from build123d import *

# Parameters (mm, degrees)
SKETCH1_W           = 74.93
SKETCH1_H           = 34.036
BOSS_EXTRUDE1_DEPTH = 16.002
FILLET1_R           = 9.525
SKETCH2_R           = 2.54
BOSS_EXTRUDE2_DEPTH = 25.4
FILLET2_R           = 2.6035


with BuildPart() as part:
    # Sketch1 → Boss-Extrude1 (new body)
    with BuildSketch(Plane.XY):
        with Locations((37.465, 17.018)):
            Rectangle(SKETCH1_W, SKETCH1_H)
    extrude(amount=BOSS_EXTRUDE1_DEPTH)

    # Fillet1
    # the kernel refuses this fillet: 9.525 mm, written as the material it takes off along each edge
    with BuildSketch(Plane(origin=(74.93, -23.8125, 16.002), x_dir=(0, 0, -1), z_dir=(0, 1, 0))) as fillet1_piece_1:
        with BuildLine():
            CenterArc((FILLET1_R, FILLET1_R), FILLET1_R, 180, 90)
            Line((0, FILLET1_R), (0, 0))
            Line((0, 0), (FILLET1_R, 0))
        make_face()
    extrude(amount=81.661, mode=Mode.SUBTRACT)
    with BuildSketch(Plane(origin=(74.93, -23.8125, 0), x_dir=(0, 0, 1), z_dir=(0, 1, 0))) as fillet1_piece_2:
        with BuildLine():
            CenterArc((FILLET1_R, -FILLET1_R), FILLET1_R, 90, 90)
            Line((0, -FILLET1_R), (0, 0))
            Line((0, 0), (FILLET1_R, 0))
        make_face()
    extrude(amount=81.661, mode=Mode.SUBTRACT)

    # Sketch2 → Boss-Extrude2 (add)
    with BuildSketch(Plane(origin=(0, 34.036, 0), x_dir=(1, 0, 0), z_dir=(0, 1, 0))):
        with Locations(Location((67.187289562, -4.5085, 0), (0, 0, 90))):
            Circle(SKETCH2_R)
        with Locations(Location((67.187289562, -11.4935, 0), (0, 0, 90))):
            Circle(SKETCH2_R)
    extrude(amount=BOSS_EXTRUDE2_DEPTH)

    # Fillet2
    fillet2_edges = [part.edges().sort_by_distance(p)[0] for p in [
        (0, 17.018, 16.002),
        (0, 17.018, 0),
        (0, 34.036, 8.001),
        (0, 0, 8.001),
    ]]
    fillet(fillet2_edges, radius=FILLET2_R)


solid = part.part
Work out the finished part from the listing and answer in its coordinate system (mm). A direction names the side the tool comes from. Give positions to 0.01 mm unless a question says otherwise; leave off trailing zeros. Loops run counter-clockwise (first coordinate to the right, second up) from the corner with the lowest first, then second, coordinate; pieces in that order, holes last. Notation, with made-up numbers: (8, -4) -> (34, -4) arc R35 cw to (34, 28) -> close; hole circle Ø3 at (18.5, -29.75). An arc over 180 degrees is marked (long way). Use a Markdown table: item, result. Add a question column.
1) Each of these flat-tipped pins is pushed along its axis until it touches: P1, Ø4, axis at x = 42.5, z = 7.5, coming from the -Y side; P2, Ø2, axis at x = 27, z = 7.5, coming from the +Y side; P3, Ø6, axis at y = 30, z = 3.5, coming from the +X side. Where does it stop, or does it pass through?
2) Consider line 1 along Z through (x, y) = (67, 40.5); line 2 along Y through (x, z) = (37.5, 1.75); line 3 along X through (y, z) = (10, 12.25). Determine where each line is inside the solid, lowest interval first.
3) Which of the six approach directions +Z, -Z, +X, -X, +Y, -Y give full straight-line access (tool end or side, diameter ignored) to faces 1 (the cylindrical face through (67.08, 46.56, 14.03)), 2 (the cylindrical face through (0.742, 17.256, 0.783))?
4) For a pull along Z with two mould halves and no side action, classify faces 3 (the cylindrical face through (0.742, 0.783, 8.113)), 4 (the flat face through (34, 17, 16.002)), 5 (the flat face through (34, 17, 0)), 6 (the cylindrical face through (64.67, 46.56, 4.84)) as +Z half, -Z half, draft (parallel to the pull), parting line (faces both ways), or undercut.
5) The part is cut by section B-B, the plane z = 5.5. Determine the outline of the cut face in (x, y), plus the area to 3 significant figures.
6) The part is cut by section C-C, the plane x = 55. Determine the outline of the cut face in (y, z), plus the area to 3 significant figures.
7) The part is cut by section D-D, the plane y = 50. Determine the outline of the cut face in (x, z).
Reported:
| question | item | result |
|---|---|---|
| 1 | P1 | stops at y = 0 |
| 1 | P2 | stops at y = 34.04 |
| 1 | P3 | stops at x = 74.44 |
| 2 | line 1 | z = 1.98 to 7.04, 8.96 to 14.03 |
| 2 | line 2 | y = 0 to 34.04 |
| 2 | line 3 | x = 0 to 72.98 |
| 3 | face 1 | +Y |
| 3 | face 2 | -Z, -X, +Y, -Y |
| 4 | face 3 | draft |
| 4 | face 4 | +Z half |
| 4 | face 5 | -Z half |
| 4 | face 6 | undercut |
| 5 | outline | (0, 2.6) arc R2.6 ccw to (2.6, 0) -> (74.04, 0) -> (74.04, 34.04) -> (69.53, 34.04) -> (69.53, 59.44) -> (64.85, 59.44) -> (64.85, 34.04) -> (2.6, 34.04) arc R2.6 ccw to (0, 31.43) -> close |
| 5 | area | 2,640 mm^2 |
| 6 | outline | (0, 0) -> (34.04, 0) -> (34.04, 16) -> (0, 16) -> close |
| 6 | area | 545 mm^2 |
| 7 | outline | circle Ø5.08 at (67.19, 4.51); circle Ø5.08 at (67.19, 11.49) |
